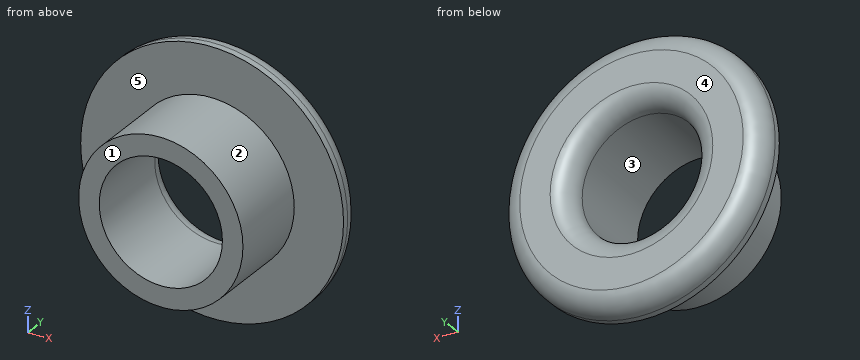
```python
from build123d import *

# Parameters (mm, degrees)
SKETCH1_R           = 3.175
SKETCH1_R_2         = 2.38125
BOSS_EXTRUDE1_DEPTH = 3.175
SKETCH2_R           = 5.08
SKETCH2_R_2         = 2.38125
BOSS_EXTRUDE2_DEPTH = 1.016
FILLET1_R           = 0.762


with BuildPart() as part:
    # Sketch1 → Boss-Extrude1 (new body)
    with BuildSketch(Plane(origin=(0, 0, 0), x_dir=(1, 0, 0), z_dir=(0, 1, 0))):
        Circle(SKETCH1_R)
        Circle(SKETCH1_R_2, mode=Mode.SUBTRACT)
    extrude(amount=BOSS_EXTRUDE1_DEPTH)

    # Sketch2 → Boss-Extrude2 (add)
    with BuildSketch(Plane(origin=(0, 3.175, 0), x_dir=(1, 0, 0), z_dir=(0, 1, 0))):
        Circle(SKETCH2_R)
        Circle(SKETCH2_R_2, mode=Mode.SUBTRACT)
    extrude(amount=BOSS_EXTRUDE2_DEPTH)

    # Fillet1
    fillet1_edges = [part.edges().sort_by_distance(p)[0] for p in [
        (-2.38125, 4.191, 0),
        (-5.08, 4.191, 0),
    ]]
    fillet(fillet1_edges, radius=FILLET1_R)


solid = part.part
```
Read the model definition and answer for the solid it produces. Units are mm, in the model's axes. Face numbers are marked on the shaded views. A direction names the side the tool comes from. Round coordinates to 2 decimals unless told otherwise and drop trailing zeros. Write each loop counter-clockwise with the first axis right and the second up, starting at its lowest first coordinate (ties: lowest second). Pieces come first, ordered by that corner, then holes. Notation, with made-up numbers: (26.5, -19.75) -> (40.5, -19.75) arc R22 ccw to (40.5, -9.75) -> close; hole circle Ø10 at (49.25, -32). An arc over 180 degrees is marked (long way). Answer in a Markdown table with one row per item. Add a question column.
1) Find section D-D, the plane y = 3.85. Determine the outline of the cut face in (x, z).
2) Given P1, Ø1, axis at x = 3, y = 1, coming from the +Z side; P2, Ø5.5, axis at x = 0, z = 0, coming from the +Y side, each flat-ended and moving along its own axis, determine where each tip first touches the part or whether it passes through.
3) Find section B-B, the plane x = 0. Determine the outline of the cut face in (y, z) (3 decimals).
4) Find section A-A, the plane z = 0. Determine the outline of the cut face in (x, y) (3 decimals).
5) Consider line 1 (X direction, y = 2.25, z = 0) (3 decimals); line 2 (Y direction, x = 0.25, z = 4) (3 decimals). Determine where each line is inside the solid, lowest interval first.
6) Which of the six approach directions +Z, -Z, +X, -X, +Y, -Y give full straight-line access (tool end or side, diameter ignored) to the marked faces 4 and 5?
7) Determine the mould class of the marked faces 1, 2 and 3 for opening direction X: pulls with the +X half, pulls with the -X half, needs draft (parallel to the pull), parting line crosses it, or undercut.
Findings below:
| question | item | result |
|---|---|---|
| 1 | outline | circle Ø9.91 at (0, 0); hole circle Ø5.02 at (0, 0) |
| 2 | P1 | z = 1.96 |
| 2 | P2 | y = 4.08 |
| 3 | outline | (0, -3.175) -> (3.175, -3.175) -> (3.175, -5.08) -> (3.429, -5.08) arc R0.762 ccw to (4.191, -4.318) -> (4.191, -3.143) arc R0.762 ccw to (3.429, -2.381) -> (0, -2.381) -> close; (0, 2.381) -> (3.429, 2.381) arc R0.762 ccw to (4.191, 3.143) -> (4.191, 4.318) arc R0.762 ccw to (3.429, 5.08) -> (3.175, 5.08) -> (3.175, 3.175) -> (0, 3.175) -> close |
| 4 | outline | (-5.08, 3.175) -> (-3.175, 3.175) -> (-3.175, 0) -> (-2.381, 0) -> (-2.381, 3.429) arc R0.762 ccw to (-3.143, 4.191) -> (-4.318, 4.191) arc R0.762 ccw to (-5.08, 3.429) -> close; (2.381, 0) -> (3.175, 0) -> (3.175, 3.175) -> (5.08, 3.175) -> (5.08, 3.429) arc R0.762 ccw to (4.318, 4.191) -> (3.143, 4.191) arc R0.762 ccw to (2.381, 3.429) -> close |
| 5 | line 1 | -3.175 to -2.381, 2.381 to 3.175 |
| 5 | line 2 | 3.175 to 4.191 |
| 6 | face 4 | +Z, -Z, +X, -X, +Y |
| 6 | face 5 | -Y |
| 7 | face 1 | needs draft |
| 7 | face 2 | parting line crosses it |
| 7 | face 3 | undercut |
